from build123d import *

# Parameters (mm, degrees)
SKETCH1_R           = 2.413
BOSS_EXTRUDE1_DEPTH = 3.175
FILLET1_R           = 10
CUT_EXTRUDE1_REACH  = 5.175
SKETCH2_W           = 3.175
SKETCH2_H           = 31.75


with BuildPart() as part:
    # Sketch1 → Boss-Extrude1 (new body)
    with BuildSketch(Plane(origin=(0, 0, 0), x_dir=(1, 0, 0), z_dir=(0, 1, 0))):
        with BuildLine():
            ThreePointArc((-18.288, -16.933333333), (0, -35.221333333), (18.288, -16.933333333))
            Line((18.288, -16.933333333), (18.288, -4.325934222))
            Line((18.288, -4.325934222), (36.593688296, 32.202894511))
            ThreePointArc((36.593688296, 32.202894511), (35.804843833, 50.003854168), (20.2438, 58.6843124))
            Line((20.2438, 58.6843124), (-20.2438, 58.6843124))
            ThreePointArc((-20.2438, 58.6843124), (-35.804843833, 50.003854168), (-36.593688296, 32.202894511))
            Line((-36.593688296, 32.202894511), (-18.288, -4.325934222))
            Line((-18.288, -4.325934222), (-18.288, -16.933333333))
        make_face()
        Circle(SKETCH1_R, mode=Mode.SUBTRACT)
        with Locations((0, -16.933333333)):
            Circle(SKETCH1_R, mode=Mode.SUBTRACT)
        with Locations((-20.2438, 40.3963124)):
            Circle(SKETCH1_R, mode=Mode.SUBTRACT)
        with Locations((20.2438, 40.3963124)):
            Circle(SKETCH1_R, mode=Mode.SUBTRACT)
    extrude(amount=BOSS_EXTRUDE1_DEPTH)

    # Fillet1
    fillet1_edges = [part.edges().sort_by_distance(p)[0] for p in [
        (-18.288, 1.5875, 4.325934222),
        (18.288, 1.5875, 4.325934222),
    ]]
    fillet(fillet1_edges, radius=FILLET1_R)

    # Sketch2 → Cut-Extrude1 (cut, up to next)
    with BuildSketch(Plane(origin=(0, 3.175, 0), x_dir=(1, 0, 0), z_dir=(0, 1, 0)), mode=Mode.PRIVATE) as cut_extrude1_sk1:
        with Locations((-7.9375, 12.1134886)):
            Rectangle(SKETCH2_W, SKETCH2_H)
    cut_extrude1_tool1 = extrude(cut_extrude1_sk1.sketch, amount=-CUT_EXTRUDE1_REACH, mode=Mode.PRIVATE) & part.part
    add(cut_extrude1_tool1.solids().sort_by_distance((-7.9375, 3.175, -12.113489))[0], mode=Mode.SUBTRACT)
    # Sketch2 → Cut-Extrude1 (cut, up to next)
    with BuildSketch(Plane(origin=(0, 3.175, 0), x_dir=(1, 0, 0), z_dir=(0, 1, 0)), mode=Mode.PRIVATE) as cut_extrude1_sk2:
        with Locations((7.9375, 12.1134886)):
            Rectangle(SKETCH2_W, SKETCH2_H)
    cut_extrude1_tool2 = extrude(cut_extrude1_sk2.sketch, amount=-CUT_EXTRUDE1_REACH, mode=Mode.PRIVATE) & part.part
    add(cut_extrude1_tool2.solids().sort_by_distance((7.9375, 3.175, -12.113489))[0], mode=Mode.SUBTRACT)


solid = part.part
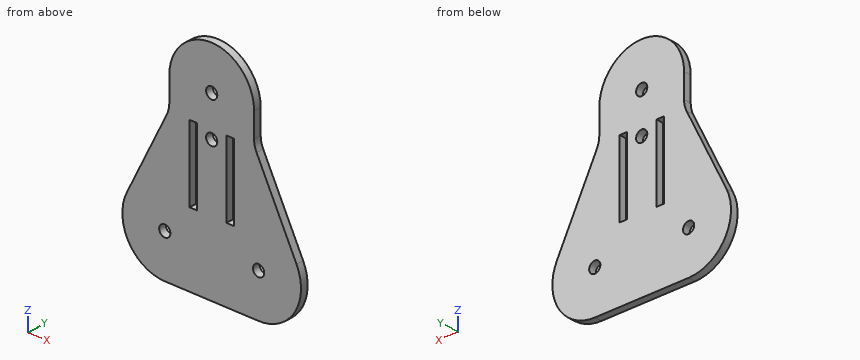
For this review, take the finished solid that the model builds, in its own axes (mm). Give positions to 0.01 mm unless a question says otherwise; leave off trailing zeros. Loops run counter-clockwise (first coordinate to the right, second up) from the corner with the lowest first, then second, coordinate; pieces in that order, holes last. Notation, with made-up numbers: (35, 57) - (50, 57) arc R12 ccw to (50, 72) - close; hole circle Ø7 at (53.5, 51.25). An arc over 180 degrees is marked (long way). Write each question's results on one line, items separated by ' | '.
(1) Take a section at D-D (y = 1.2). Give the boundary of the cut face in (x, z) (3 decimals).
Conclusion:
outline: (-36.594, -32.203) arc R18.288 ccw to (-20.244, -58.684) - (20.244, -58.684) arc R18.288 ccw to (36.594, -32.203) - (19.348, 2.211) arc R10 cw to (18.288, 6.691) - (18.288, 16.933) arc R18.288 ccw to (-18.288, 16.933) - (-18.288, 6.691) arc R10 cw to (-19.348, 2.211) - close; hole circle Ø4.826 at (-20.244, -40.396); hole (-9.525, -27.988) - (-6.35, -27.988) - (-6.35, 3.762) - (-9.525, 3.762) - close; hole circle Ø4.826 at (0, 0); hole circle Ø4.826 at (0, 16.933); hole (6.35, -27.988) - (9.525, -27.988) - (9.525, 3.762) - (6.35, 3.762) - close; hole circle Ø4.826 at (20.244, -40.396)
(2) Take a section at B-B (z = 0). Give the boundary of the cut face in (x, y) (3 decimals), then the cut area to 3 significant figures.
Conclusion:
outline: (-20.456, 0) - (-9.525, 0) - (-9.525, 3.175) - (-20.456, 3.175) - close; (-6.35, 0) - (-2.413, 0) - (-2.413, 3.175) - (-6.35, 3.175) - close; (2.413, 0) - (6.35, 0) - (6.35, 3.175) - (2.413, 3.175) - close; (9.525, 0) - (20.456, 0) - (20.456, 3.175) - (9.525, 3.175) - close | area: 94.4 mm^2
(3) Take a section at A-A (x = 0). Give the boundary of the cut face in (y, z) (3 decimals).
Conclusion:
outline: (0, -58.684) - (3.175, -58.684) - (3.175, -2.413) - (0, -2.413) - close; (0, 2.413) - (3.175, 2.413) - (3.175, 14.52) - (0, 14.52) - close; (0, 19.346) - (3.175, 19.346) - (3.175, 35.221) - (0, 35.221) - close
(4) Take a section at C-C (z = -23). Give the boundary of the cut face in (x, y) (3 decimals).
Conclusion:
outline: (-31.982, 0) - (-9.525, 0) - (-9.525, 3.175) - (-31.982, 3.175) - close; (-6.35, 0) - (6.35, 0) - (6.35, 3.175) - (-6.35, 3.175) - close; (9.525, 0) - (31.982, 0) - (31.982, 3.175) - (9.525, 3.175) - close
(5) For pin 1 Ø1 at (y, z) = (1, 11.5) entering from +X; pin 2 Ø1.5 at (x, z) = (-17.5, 1) entering from -Y; pin 3 Ø1 at (x, y) = (-7.5, 2) entering from +Z; pin 4 Ø1 at (y, z) = (1.5, -7.5) entering from -X, all flat-tipped, find the tip position at first contact; note any pin that passes through.
Conclusion:
pin 1: x = 18.29 | pin 2: y = 0 | pin 3: z = 33.83 | pin 4: x = -24.46
(6) For line 1 along Z through (x, y) = (0, 1.4); line 2 along X through (y, z) = (2.15, -23.5) (3 decimals); line 3 along X through (y, z) = (2.55, 0) (3 decimals), list the stretches that pass through material, from the lowest coordinate up.
Conclusion:
line 1: -58.68 to -2.41, 2.41 to 14.52, 19.35 to 35.22 | line 2: -32.232 to -9.525, -6.35 to 6.35, 9.525 to 32.232 | line 3: -20.456 to -9.525, -6.35 to -2.413, 2.413 to 6.35, 9.525 to 20.456
